Geometry check sheet. Reference: the model listing, model coordinates, mm. Face numbers are marked on the shaded views. A direction names the side the tool comes from. Coordinates: 2 decimals unless noted, no trailing zeros. Write each loop counter-clockwise with the first axis right and the second up, starting at its lowest first coordinate (ties: lowest second). Pieces come first, ordered by that corner, then holes. Notation, with made-up numbers: (-8.75, 83) -> (-1.75, 83) arc R35 ccw to (-1.75, 121) -> close; hole circle Ø10 at (35, 86). An arc over 180 degrees is marked (long way). One line per question, with ' | ' between items.
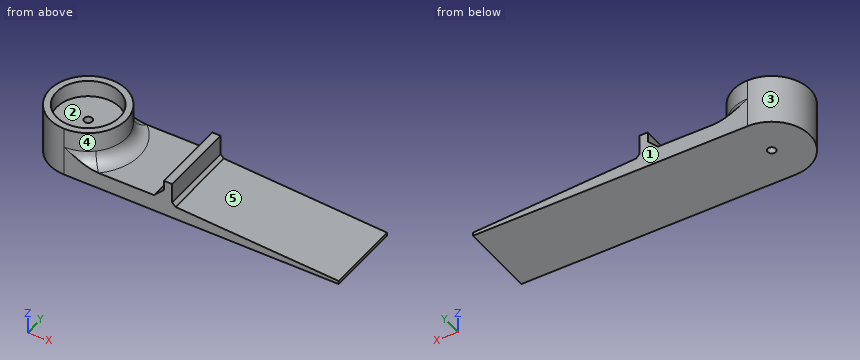
```python
from build123d import *

# Parameters (mm, degrees)
PAD_DEPTH       = 11.5
POCKET_DEPTH    = 15
SKETCH003_R     = 9.5
POCKET001_DEPTH = 5
POCKET002_DEPTH = 10
FILLET_R        = 4
CHAMFER_SIZE    = 3
CHAMFER001_SIZE = 1
SKETCH006_R     = 1.25
POCKET003_DEPTH = 30


with BuildPart() as part:
    # Sketch → Pad (new body, symmetric)
    with BuildSketch(Plane.XZ):
        Polygon((-11.5, 0), (82.5, 0), (82.5, 1), (32.5, 4), (32.5, 11), (30, 11), (30, 5), (11.5, 5), (11.5, 15), (-11.5, 15), align=None)
    extrude(amount=PAD_DEPTH, both=True)

    # Sketch001 → Pocket (cut)
    with BuildSketch(Plane.XY):
        with BuildLine():
            ThreePointArc((-0.035747, 11.499944), (-11.5, 0), (-0.035747, -11.499944))
            Line((-0.035747, -11.499944), (-0.035747, -22.999972))
            ThreePointArc((-0.035747, 22.999972), (-23, 0), (-0.035747, -22.999972))
            Line((-0.035747, 22.999972), (-0.035747, 11.499944))
        make_face()
    extrude(amount=POCKET_DEPTH, mode=Mode.SUBTRACT)

    # Sketch003 (on DatumPlane) → Pocket001 (cut)
    with BuildSketch(Plane(origin=(0, 0, 15), x_dir=(-1, 0, 0), z_dir=(0, 0, 1))):
        Circle(SKETCH003_R)
    extrude(amount=-POCKET001_DEPTH, mode=Mode.SUBTRACT)

    # Sketch005 (on Face1 of Pocket001) → Pocket002 (cut)
    with BuildSketch(Plane(origin=(0, 0, 15), x_dir=(-1, 0, 0), z_dir=(0, 0, 1))):
        with BuildLine():
            ThreePointArc((0, 11.5), (-11.5, 0), (0, -11.5))
            Line((0, -11.5), (0, -23))
            ThreePointArc((0, 23), (-23, 0), (0, -23))
            Line((0, 23), (0, 11.5))
        make_face()
    extrude(amount=-POCKET002_DEPTH, mode=Mode.SUBTRACT)

    # Fillet
    fillet_edges = [part.edges().sort_by_distance(p)[0] for p in [
        (8.131728, -8.131728, 5),
        (8.131728, 8.131728, 5),
    ]]
    fillet(fillet_edges, radius=FILLET_R)

    # Chamfer
    chamfer_edges = [part.edges().sort_by_distance(p)[0] for p in [
        (30, 0, 5),
    ]]
    chamfer(chamfer_edges, length=CHAMFER_SIZE)

    # Chamfer001
    chamfer001_edges = [part.edges().sort_by_distance(p)[0] for p in [
        (32.5, 0, 4),
    ]]
    chamfer(chamfer001_edges, length=CHAMFER001_SIZE)

    # Sketch006 → Pocket003 (cut)
    with BuildSketch(Plane.XY):
        Circle(SKETCH006_R)
    extrude(amount=POCKET003_DEPTH, mode=Mode.SUBTRACT)


solid = part.part
```
(1) Cross-section at D-D (x = 41.5). Record the cut outline in (y, z).
Answers below:
outline: (-11.5, 0) -> (11.5, 0) -> (11.5, 3.46) -> (-11.5, 3.46) -> close
(2) Material ranges on line 1 (X direction, y = 0, z = 13.8); line 2 (X direction, y = 0, z = 5.75); line 3 (X direction, y = 0, z = 5.5), recorded low to high.
Answers below:
line 1: x = -11.5 to -9.5, 9.5 to 11.5 | line 2: x = -11.5 to -1.25, 1.25 to 13.17, 27.75 to 32.5 | line 3: x = -11.5 to -1.25, 1.25 to 13.56, 27.5 to 32.5
(3) Draft check along X on the marked faces 3, 4 and 5. Enter one of: pulls with the +X half, pulls with the -X half, needs draft (parallel to the pull), parting line crosses it, or undercut.
Answers below:
face 3: pulls with the -X half | face 4: undercut | face 5: pulls with the +X half
(4) Tool access check on the marked faces 1 and 2. Record the directions out of +Z, -Z, +X, -X, +Y, -Y that give a thin tool (end or side, any length) a straight path to the whole face; none if there is none.
Answers below:
face 1: +Z, -Z, +X, -X, +Y | face 2: +Z
(5) Cross-section at A-A (y = 0). Record the cut outline in (x, z), plus the area to 3 significant figures.
Answers below:
outline: (-11.5, 0) -> (-1.25, 0) -> (-1.25, 10) -> (-9.5, 10) -> (-9.5, 15) -> (-11.5, 15) -> close; (1.25, 0) -> (82.5, 0) -> (82.5, 1) -> (33.5, 3.94) -> (32.5, 5) -> (32.5, 11) -> (30, 11) -> (30, 8) -> (27, 5) -> (15.5, 5) arc R4 cw to (11.5, 9) -> (11.5, 15) -> (9.5, 15) -> (9.5, 10) -> (1.25, 10) -> close | area: 478 mm²
(6) Depth check by flat-ended pin: P1, Ø0.8, axis at x = 31.5, y = 5, coming from the +Z side; P2, Ø1.5, axis at y = -4, z = 9, coming from the -X side; P3, Ø1, axis at x = 1, z = 11.5, coming from the -Y side. Enter the tip coordinate at first touch or a pass-through.
Answers below:
P1: stops at z = 11 | P2: stops at x = -11.03 | P3: stops at y = -11.49
(7) Cross-section at B-B (x = 68). Record the cut outline in (y, z).
Answers below:
outline: (-11.5, 0) -> (11.5, 0) -> (11.5, 1.87) -> (-11.5, 1.87) -> close
